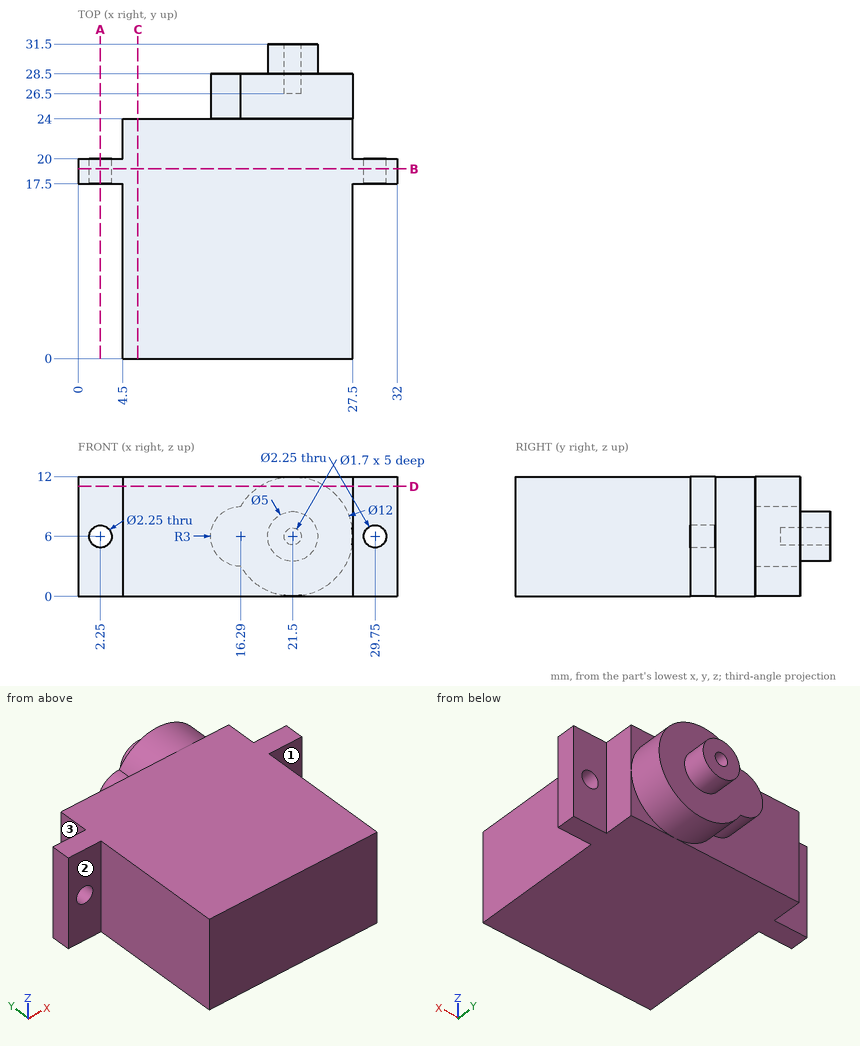
For this review, use the dimensioned drawing (mm, ordinates from the lowest corner) and the shaded views. A direction names the side the tool comes from. Give positions to 0.01 mm unless a question says otherwise; leave off trailing zeros. Write each loop counter-clockwise with the first axis right and the second up, starting at its lowest first coordinate (ties: lowest second). Pieces come first, ordered by that corner, then holes. Notation, with made-up numbers: M 72.25,30 L 94.25,30 A22 cw 94.25,67 Z; hole C 69,30 d9. An arc over 180 degrees is marked long. Answer as a JSON object with one key per item and string values. Group by question number.
Item 1: Consider section D-D on z = 11. Write out the cut boundary in (x, y).
Item 2: Tool access review of the marked faces 1, 2 and 3: name each direction out of +Z, -Z, +X, -X, +Y, -Y from which nothing blocks a thin tool from reaching the whole face with its end or side.
Item 3: Consider section A-A on x = 2.25. Write out the cut boundary in (y, z) (3 decimals).
Item 4: For probe 1 along X at (y, z) = (18.6, 6) (3 decimals); probe 2 along X at (y, z) = (27.65, 6); probe 3 along Y at (x, z) = (4, 11.25), list the stretches that pass through material, from the lowest coordinate up. Write a range as [from, to].
Item 5: Consider section C-C on x = 6. Write out the cut boundary in (y, z), plus the area to 3 significant figures.
Item 6: Consider section B-B on y = 19. Write out the cut boundary in (x, z) (3 decimals), plus the area to 3 significant figures.
Item 7: For pin 1 Ø3.5 at (x, z) = (3, 5.5) entering from +Y; pin 2 Ø4.5 at (y, z) = (22, 6.5) entering from -X; pin 3 Ø1.3 at (x, z) = (30.5, 4.5) entering from -Y; pin 4 Ø1.5 at (y, z) = (25, 10) entering from -X, all flat-tipped, find the tip position at first contact; note any pin that passes through.
Check result:
{
 "1": {"outline": "M 0,17.5 L 4.5,17.5 L 4.5,0 L 27.5,0 L 27.5,17.5 L 32,17.5 L 32,20 L 27.5,20 L 27.5,24 L 24.82,24 L 24.82,28.5 L 18.18,28.5 L 18.18,24 L 4.5,24 L 4.5,20 L 0,20 Z"},
 "2": {"face 1": "+Z, -Z, +X, -Y", "face 2": "+Z, -Z, -X, -Y", "face 3": "+Z, -Z, -X, +Y"},
 "3": {"outline": "M 17.5,0 L 20,0 L 20,4.875 L 17.5,4.875 Z; M 17.5,7.125 L 20,7.125 L 20,12 L 17.5,12 Z"},
 "4": {"probe 1": "x = [0, 1.125], [3.375, 28.625], [30.875, 32]", "probe 2": "x = [13.29, 20.65], [22.35, 27.5]", "probe 3": "y = [17.5, 20]"},
 "5": {"outline": "M 0,0 L 24,0 L 24,12 L 0,12 Z", "area": "288 mm^2"},
 "6": {"outline": "M 0,0 L 32,0 L 32,12 L 0,12 Z; hole C 2.25,6 d2.25; hole C 29.75,6 d2.25", "area": "376 mm^2"},
 "7": {"pin 1": "stops at y = 24", "pin 2": "stops at x = 0", "pin 3": "stops at y = 17.5", "pin 4": "stops at x = 16.46"}
}
